from build123d import *

# Parameters (mm, degrees)
SKETCH1_R           = 35
SKETCH1_R_2         = 20
BOSS_EXTRUDE1_DEPTH = 7.5
SKETCH2_R           = 32.5
SKETCH2_R_2         = 22.5
CUT_EXTRUDE1_DEPTH  = 1


with BuildPart() as part:
    # Sketch1 → Boss-Extrude1 (new body, symmetric)
    with BuildSketch(Plane.XY):
        Circle(SKETCH1_R)
        Circle(SKETCH1_R_2, mode=Mode.SUBTRACT)
    extrude(amount=BOSS_EXTRUDE1_DEPTH, both=True)

    # Sketch2 → Cut-Extrude1 (cut)
    with BuildSketch(Plane.XY.offset(7.5)):
        Circle(SKETCH2_R)
        Circle(SKETCH2_R_2, mode=Mode.SUBTRACT)
    cut_extrude1 = extrude(amount=-CUT_EXTRUDE1_DEPTH, mode=Mode.SUBTRACT)

    # Mirror1: Cut-Extrude1 across plane
    add(cut_extrude1.mirror(Plane.XY), mode=Mode.SUBTRACT)


solid = part.part
CAD build for the part. Positions are in the model's coordinates, mm. A direction names the side the tool comes from. Give positions to 0.01 mm unless a question says otherwise; leave off trailing zeros. Write each loop counter-clockwise with the first axis right and the second up, starting at its lowest first coordinate (ties: lowest second). Pieces come first, ordered by that corner, then holes. Notation, with made-up numbers: (-36, 61) - (-23, 61) arc R26 ccw to (-23, 84) - close; hole circle Ø10 at (8, 78.5). An arc over 180 degrees is marked (long way). Answer as CSV lines item,"result".
Q1. Drill centre lines: line 1 (Y direction, x = 0, z = 7.05); line 2 (Y direction, x = 0, z = 1.75); line 3 (Z direction, x = 14.5, y = -18). Where is each one in solid material? Low to high. Write a range as from..to.
Result set:
line 1,"-35..-32.5, -22.5..-20, 20..22.5, 32.5..35"
line 2,"-35..-20, 20..35"
line 3,"-6.5..6.5"
Q2. Band-saw the part on A-A (x = 0). Give the cut face in (y, z), and give its area (3 significant figures).
Result set:
outline,"(-35, -7.5) - (-32.5, -7.5) - (-32.5, -6.5) - (-22.5, -6.5) - (-22.5, -7.5) - (-20, -7.5) - (-20, 7.5) - (-22.5, 7.5) - (-22.5, 6.5) - (-32.5, 6.5) - (-32.5, 7.5) - (-35, 7.5) - close; (20, -7.5) - (22.5, -7.5) - (22.5, -6.5) - (32.5, -6.5) - (32.5, -7.5) - (35, -7.5) - (35, 7.5) - (32.5, 7.5) - (32.5, 6.5) - (22.5, 6.5) - (22.5, 7.5) - (20, 7.5) - close"
area,"410 mm²"
Q3. Flat gauge pins, fed straight in: pin 1 Ø2 at (x, z) = (-7, -1) entering from +Y; pin 2 Ø4 at (x, y) = (27.5, 1.5) entering from -Z; pin 3 Ø1 at (y, z) = (-7.5, 4.5) entering from +X. Where does each tip first touch, or does it go through?
Result set:
pin 1,"y = 34.48"
pin 2,"z = -6.5"
pin 3,"x = 34.29"
Q4. Band-saw the part on D-D (z = 2.5). Give the cut face in (x, y).
Result set:
outline,"circle Ø70 at (0, 0); hole circle Ø40 at (0, 0)"
Q5. Band-saw the part on C-C (x = 28). Give the cut face in (y, z).
Result set:
outline,"(-21, -7.5) - (-16.5, -7.5) - (-16.5, -6.5) - (16.5, -6.5) - (16.5, -7.5) - (21, -7.5) - (21, 7.5) - (16.5, 7.5) - (16.5, 6.5) - (-16.5, 6.5) - (-16.5, 7.5) - (-21, 7.5) - close"
Q6. 3-axis set-ups, long thin cutter, end or side, ignore diameter. For faces 1 (the face through (10.382, -19.961, -7.007)), 2 (the face through (-4.336, -19.524, -0.105)), 3 (the face through (10.382, -19.961, 7.007)): which of +Z, -Z, +X, -X, +Y, -Y reach the whole face in a straight line?
Result set:
face 1,"-Z"
face 2,"+Z, -Z"
face 3,"+Z"
Q7. Pull direction X, two halves, no side cores. Call faces 4 (the face through (31, 9.76, -7.01)), 5 (the face through (-28, -21, 0)), 6 (the face through (-20.1, -1.6, -7.5)): released by +X, released by -X, zero draft, split by the parting line, or undercut.
Result set:
face 4,"undercut"
face 5,"split by the parting line"
face 6,"zero draft"
